Could you check a few things on this model? Use its own coordinates, in mm. Face numbers are marked on the shaded views. A direction names the side the tool comes from. Round coordinates to 2 decimals unless told otherwise and drop trailing zeros. Loops run counter-clockwise (first coordinate to the right, second up) from the corner with the lowest first, then second, coordinate; pieces in that order, holes last. Notation, with made-up numbers: M 42,27 L 72,27 A11 cw 72,38 Z; hole C 72.5,13.5 d8. An arc over 180 degrees is marked long. Return JSON: item names as keys, results as strings. Group by question number.
```python
from build123d import *

# Parameters (mm, degrees)
SKETCH_R     = 5
PAD_DEPTH    = 6
POCKET_DEPTH = 4
SKETCH002_R  = 3
PAD001_DEPTH = 20
FILLET_R     = 0.5
CHAMFER_SIZE = 0.5


with BuildPart() as part:
    # Sketch → Pad (new body)
    with BuildSketch(Plane.XY):
        Circle(SKETCH_R)
    extrude(amount=PAD_DEPTH)

    # Sketch001 (on Face3 of Pad) → Pocket (cut)
    with BuildSketch(Plane.XY.offset(6)):
        Polygon((2.886751, 0), (1.443376, 2.5), (-1.443376, 2.5), (-2.886751, 0), (-1.443376, -2.5), (1.443376, -2.5), align=None)
    extrude(amount=-POCKET_DEPTH, mode=Mode.SUBTRACT)

    # Sketch002 → Pad001 (join)
    with BuildSketch(Plane.XY):
        Circle(SKETCH002_R)
    extrude(amount=-PAD001_DEPTH)

    # Fillet
    fillet_edges = [part.edges().sort_by_distance(p)[0] for p in [
        (-5, 0, 6),
    ]]
    fillet(fillet_edges, radius=FILLET_R)

    # Chamfer
    chamfer_edges = [part.edges().sort_by_distance(p)[0] for p in [
        (-3, 0, -20),
    ]]
    chamfer(chamfer_edges, length=CHAMFER_SIZE)


solid = part.part
```
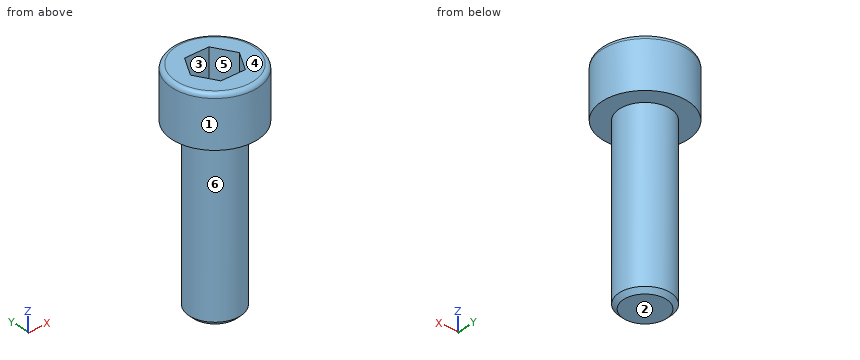
1. If we section it at A-A, the plane x = 0: Please give me the cut outline in (y, z), then the cut area to 3 significant figures.
2. I'm going to push flat-ended pins straight in: pin 1 Ø2 at (y, z) = (3, -16) entering from -X; pin 2 Ø1 at (x, z) = (-4, -5) entering from -Y; pin 3 Ø4 at (x, y) = (-0.5, -1.5) entering from +Z; pin 4 Ø1.5 at (x, y) = (0, -1) entering from +Z. Where does each tip first touch, or does it pass through?
3. We'd pull the mould along Y, two halves only. Please class the marked faces 1, 2 and 3: +Y half, -Y half, draft (parallel to the pull), parting line (faces both ways), or undercut.
4. On a 3-axis mill with a long thin cutter (end or side, diameter ignored), from which of +Z, -Z, +X, -X, +Y, -Y can I reach the whole of each face in a straight line? I mean the marked faces 4, 5 and 6. Say none if no direction works.
5. I need wall thicknesses on probe 1 along Z at (x, y) = (3.5, -2.5); probe 2 along X at (y, z) = (-0.75, 4.75); probe 3 along X at (y, z) = (-1, 3). Which ranges of each line are inside material? Lowest first, please.
6. If we section it at B-B, the plane z = -4: Please give me the cut outline in (x, y), then the cut area to 3 significant figures.
Geometry results:
{
 "1": {"outline": "M -5,0 L -3,0 L -3,-19.5 L -2.5,-20 L 2.5,-20 L 3,-19.5 L 3,0 L 5,0 L 5,5.5 A0.5 ccw 4.5,6 L 2.5,6 L 2.5,2 L -2.5,2 L -2.5,6 L -4.5,6 A0.5 ccw -5,5.5 Z", "area": "160 mm^2"},
 "2": {"pin 1": "x = -2.24", "pin 2": "through", "pin 3": "z = 6", "pin 4": "z = 2"},
 "3": {"face 1": "parting line", "face 2": "draft", "face 3": "undercut"},
 "4": {"face 4": "+Z, +X, -X, +Y, -Y", "face 5": "+Z", "face 6": "-Z"},
 "5": {"probe 1": "0 to 6", "probe 2": "-4.94 to -2.45, 2.45 to 4.94", "probe 3": "-4.9 to -2.31, 2.31 to 4.9"},
 "6": {"outline": "C 0,0 d6", "area": "28.3 mm^2"}
}
